Verification items for the finished model (mm, model axes). A direction names the side the tool comes from. Round coordinates to 2 decimals unless told otherwise and drop trailing zeros. Loops run counter-clockwise (first coordinate to the right, second up) from the corner with the lowest first, then second, coordinate; pieces in that order, holes last. Notation, with made-up numbers: M 60,64.5 L 70,64.5 A24 cw 70,94.5 Z; hole C 56.25,51 d6. An arc over 180 degrees is marked long. Answer as CSV lines item,"result".
Autodesk Inventor part; units mm, degrees
ref_plane "YZ Plane" through (0, 0, 0) normal (1, 0, 0) x (0, 1, 0)
ref_plane "XZ Plane" through (0, 0, 0) normal (0, 1, 0) x (-1, 0, 0)
ref_plane "XY Plane" through (0, 0, 0) normal (0, 0, 1) x (1, 0, 0)
sketch "Skizze1" plane through (0, 0, 0) normal (0, 0, 1) x (1, 0, 0)
  line L0 (0, 0) -> (50, 0)
  line L1 (50, 0) -> (50, 15)
  line L2 (50, 15) -> (0, 15)
  line L3 (0, 15) -> (0, 0)
  dimension "d0" = 15
  dimension "d1" = 50
extrude "Extrusion1" add sketch "Skizze1" along normal blind 27
hole "Bohrung1" at (45, 10, 27) direction (0, 0, -1) diameter 3.4 end through all counterbore diameter 6.5 counterbore depth 3
hole "Bohrung2" at (5, 10, 27) direction (0, 0, -1) diameter 3.4 end through all counterbore diameter 6.5 counterbore depth 3
chamfer "Fase1" distance 0.5 angle 45 1 edges at (25, 0, 27)
sketch "Skizze2" plane through (0, 0, 0) normal (0, 0, -1) x (-1, 0, 0)
  line L0 (0, 15) -> (0, 0)
  line L1 (-50, 15) -> (0, 15)
  line L2 (-50, 0) -> (-50, 15)
  line L3 (-40, 15) -> (-10, 15)
  line L4 (-10, 15) -> (-10, 3)
  line L5 (-10, 3) -> (-40, 3)
  line L6 (-40, 3) -> (-40, 15)
  dimension "d25" = 10
  dimension "d26" = 10
  dimension "d27" = 12
extrude "Extrusion2" cut sketch "Skizze2" against normal blind 25.5
chamfer "Fase2" distance 2 angle 45 2 edges at (50, 15, 13.5) (0, 15, 13.5)
properties part number "Peripherie_Motor2_liegend"
1) Section check D-D (x = 45). Record the cut outline in (y, z), plus the area to 3 significant figures.
Here are the results:
outline,"M 0,0 L 8.3,0 L 8.3,24 L 6.75,24 L 6.75,27 L 0.5,27 L 0,26.5 Z; M 11.7,0 L 15,0 L 15,27 L 13.25,27 L 13.25,24 L 11.7,24 Z"
area,"304 mm^2"
2) Draft check along X on faces 1 (the flat face through (24.7, 2.6, 0)), 2 (the flat face through (0, 7, 13)), 3 (the flat face through (10, 9, 13)). Enter one of: +X half, -X half, draft (parallel to the pull), parting line (faces both ways), or undercut.
Here are the results:
face 1,"draft"
face 2,"-X half"
face 3,"undercut"
3) Go/stop test with flat-tipped pins: pin 1 (2 mm diameter, centred on x = 6, y = 9, fed in from +Z); pin 2 (2 mm diameter, centred on x = 5, y = 10, fed in from -Z). Record where each tip stops, or that it passes through.
Here are the results:
pin 1,"stops at z = 24"
pin 2,"passes through"
4) Section check B-B (z = 4). Record the cut outline in (x, y), plus the area to 3 significant figures.
Here are the results:
outline,"M 0,0 L 50,0 L 50,13 L 48,15 L 40,15 L 40,3 L 10,3 L 10,15 L 2,15 L 0,13 Z; hole C 5,10 d3.4; hole C 45,10 d3.4"
area,"368 mm^2"
5) Material ranges on probe 1 along X at (y, z) = (10, 25.85); probe 2 along X at (y, z) = (10, 24.9); probe 3 along X at (y, z) = (10, 14.5), recorded low to high.
Here are the results:
probe 1,"x = 0 to 1.75, 8.25 to 41.75, 48.25 to 50"
probe 2,"x = 0 to 1.75, 8.25 to 10, 40 to 41.75, 48.25 to 50"
probe 3,"x = 0 to 3.3, 6.7 to 10, 40 to 43.3, 46.7 to 50"
6) Section check C-C (y = 6). Record the cut outline in (x, z), plus the area to 3 significant figures.
Here are the results:
outline,"M 0,0 L 10,0 L 10,25.5 L 40,25.5 L 40,0 L 50,0 L 50,27 L 0,27 Z"
area,"585 mm^2"
7) Set-up check for faces 4 (the flat face through (25, 0, 13)), 5 (the cylindrical face through (48.173, 10.705, 25.479)), 6 (the flat face through (25, 9, 25.5)): record each of +Z, -Z, +X, -X, +Y, -Y from which the full face is reachable in a straight line by a thin tool's end or side.
Here are the results:
face 4,"+Z, -Z, +X, -X, -Y"
face 5,"+Z"
face 6,"-Z, +Y"
8) Section check A-A (x = 33.5). Record the cut outline in (y, z).
Here are the results:
outline,"M 0,0 L 3,0 L 3,25.5 L 15,25.5 L 15,27 L 0.5,27 L 0,26.5 Z"
